Drawing for the job (mm, zero at the part's lowest x, y, z). Round coordinates to 2 decimals unless told otherwise and drop trailing zeros. Write each loop counter-clockwise with the first axis right and the second up, starting at its lowest first coordinate (ties: lowest second). Pieces come first, ordered by that corner, then holes.
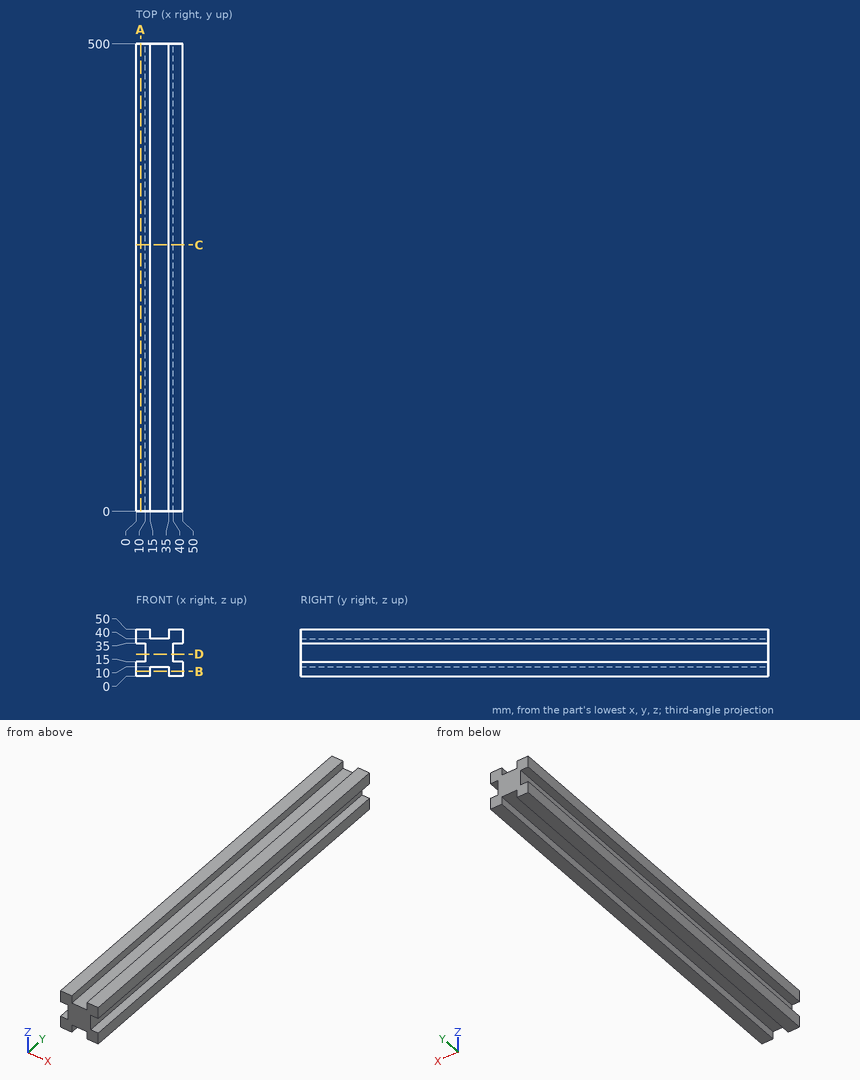
1) Cut at C-C on y = 285. List the corners of the cut face in (x, z), and give its area (3 significant figures).
2) Flat gauge pins, fed straight in: pin 1 Ø6 at (y, z) = (86.5, 24) entering from -X; pin 2 Ø16 at (y, z) = (320.5, 24) entering from +X; pin 3 Ø12 at (x, y) = (21.5, 328) entering from +Z. Where does each tip first touch, or does it go through?
3) Cut at B-B on z = 5. List the corners of the cut face in (x, y), and give its area (3 significant figures).
4) Cut at A-A on x = 5. List the corners of the cut face in (y, z), and give its area (3 significant figures).
5) Cut at D-D on z = 23.5. List the corners of the cut face in (x, y).
6) Wall check: probe 1 along X at (y, z) = (21.5, 6.5); probe 2 along Z at (x, y) = (21, 374.5). Give the ranges that are in metal, low to high.
Result sheet:
1. outline: (0, 0) - (15, 0) - (15, 10) - (35, 10) - (35, 0) - (50, 0) - (50, 15) - (40, 15) - (40, 35) - (50, 35) - (50, 50) - (35, 50) - (35, 40) - (15, 40) - (15, 50) - (0, 50) - (0, 35) - (10, 35) - (10, 15) - (0, 15) - close
1. area: 1,700 mm2
2. pin 1: stops at x = 10
2. pin 2: stops at x = 40
2. pin 3: stops at z = 40
3. outline: (0, 0) - (15, 0) - (15, 500) - (0, 500) - close; (35, 0) - (50, 0) - (50, 500) - (35, 500) - close
3. area: 15,000 mm2
4. outline: (0, 0) - (500, 0) - (500, 15) - (0, 15) - close; (0, 35) - (500, 35) - (500, 50) - (0, 50) - close
4. area: 15,000 mm2
5. outline: (10, 0) - (40, 0) - (40, 500) - (10, 500) - close
6. probe 1: x = 0 to 15, 35 to 50
6. probe 2: z = 10 to 40
